Input: part model. Units: mm. Frame: model coordinates. Face numbers are marked on the shaded views. A direction names the side the tool comes from. Coordinates: 2 decimals unless noted, no trailing zeros. Write each loop counter-clockwise with the first axis right and the second up, starting at its lowest first coordinate (ties: lowest second). Pieces come first, ordered by that corner, then holes.
1) Set-up query: the marked faces 5, 6, 7, 8 and 9. Return all of +Z, -Z, +X, -X, +Y, -Y with unobstructed straight access to the full face (end or side cutting, diameter ignored); none if empty.
2) Section query A-A (z = 2). State how many separate pieces and enclosed holes the cut face has, then the cut area to 3 significant figures.
3) Section query C-C (y = 65.75). Output: boundary loops of the cut face in (x, z), then the cut area to 3 significant figures.
4) Draft query along Y for the marked faces 1, 2, 3 and 4. Return one class per face: pulls with the +Y half, pulls with the -Y half, needs draft (parallel to the pull), parting line crosses it, or undercut.
5) Line query: L1, parallel to Z at x = 19.25, y = 55.75; L2, parallel to Z at x = 23, y = 59.5; L3, parallel to Z at x = 30, y = 65. Output: solid intervals per line, ascending.
6) Section query D-D (x = 24). Output: boundary loops of the cut face in (y, z).
7) Pin query (flat end, axial travel): pin 1 Ø0.8 at (x, y) = (29.5, 54.5) entering from -Z; pin 2 Ø6 at (x, z) = (26.5, 2) entering from +Y; pin 3 Ø4 at (x, z) = (20.5, 2) entering from +Y. Return the tip coordinate at first contact, or that it passes through.
8) Section query B-B (z = -3). Output: boundary loops of the cut face in (x, y), then the cut area to 3 significant figures.
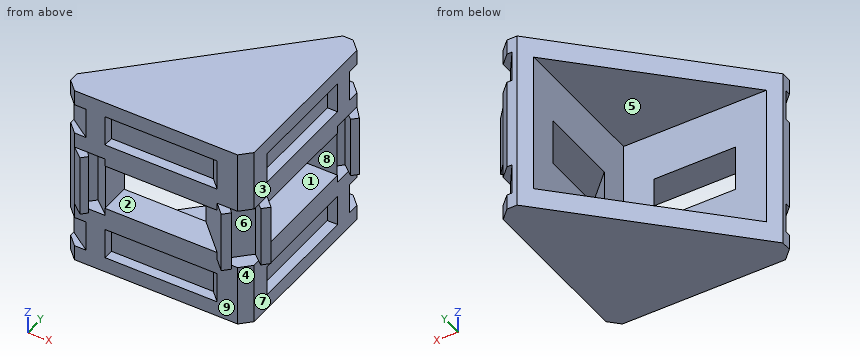
from build123d import *

# Parameters (mm, degrees)
EXTRUDE_1_DEPTH     = 6
EXTRUDE_1_2_DEPTH   = 6
EXTRUDE_1_3_DEPTH   = 6
EXTRUDE_2_DEPTH     = 4
EXTRUDE_3_DEPTH     = 2
EXTRUDE_4_DEPTH     = 0.75
EXTRUDE_5_DEPTH     = 0.75
CUT_EXTRUDE_2_DEPTH = 3
CUT_EXTRUDE_3_DEPTH = 3
CUT_EXTRUDE_4_DEPTH = 3
CUT_EXTRUDE_5_DEPTH = 3
CHAMFER_1_SIZE      = 1


with BuildPart() as part:
    # Sketch 1 → Extrude 1 (new body)
    with BuildSketch(Plane.XY):
        Polygon((32.591759834, 56.594303521), (33.206070874, 57.208614562), (29.145410702, 61.269274733), (29.145410702, 58.269274733), (26.145410702, 58.269274733), (30.206070874, 54.208614562), (30.820381914, 54.822925602), (29.852517484, 55.976381515), (31.438303921, 57.562167952), align=None)
    extrude(amount=EXTRUDE_1_DEPTH)



with BuildPart() as body_2:
    # Sketch 1 → Extrude 1 2 (new body)
    with BuildSketch(Plane.XY):
        Polygon((18.145410702, 55.352855481), (18.145410702, 58.269274733), (15.145410702, 58.269274733), (14.145410702, 57.269274733), (14.145410702, 56.269274733), (15.145410702, 55.269274733), (16.298866615, 54.301410302), (16.820381914, 54.822925602), (15.852517484, 55.976381515), (16.559624265, 56.683488296), align=None)
    extrude(amount=EXTRUDE_1_2_DEPTH)


with BuildPart() as body_3:
    # Sketch 1 → Extrude 1 3 (new body)
    with BuildSketch(Plane.XY):
        Polygon((31.438303921, 71.562167952), (32.591759834, 70.594303521), (33.113275133, 71.115818821), (32.145410702, 72.269274733), (31.145410702, 73.269274733), (30.145410702, 73.269274733), (29.145410702, 72.269274733), (29.145410702, 69.269274733), (32.061829955, 69.269274733), (30.73119714, 70.855061171), align=None)
    extrude(amount=EXTRUDE_1_3_DEPTH)


with BuildPart() as part_1:
    add(part.part)

    add(body_2.part)  # Extrude 2 merges body 2

    add(body_3.part)  # Extrude 2 merges body 3
    # Sketch 2 → Extrude 2 (add)
    with BuildSketch(Plane.XY.offset(6)):
        Polygon((30.145410702, 73.269274733), (31.145410702, 73.269274733), (32.145410702, 72.269274733), (32.145410702, 55.269274733), (15.145410702, 55.269274733), (14.145410702, 56.269274733), (14.145410702, 57.269274733), (15.145410702, 58.269274733), (29.145410702, 58.269274733), (29.145410702, 72.269274733), align=None)
    extrude_2 = extrude(amount=EXTRUDE_2_DEPTH)

    # Mirror 1: Extrude 2 across plane
    add(extrude_2.mirror(Plane(origin=(0, 0, 3), x_dir=(1, 0, 0), z_dir=(0, 0, -1))))

    # Sketch 3 → Extrude 3 (add)
    with BuildSketch(Plane.XY.offset(10)):
        Polygon((30.145410702, 73.269274733), (31.145410702, 73.269274733), (32.145410702, 72.269274733), (32.145410702, 55.269274733), (15.145410702, 55.269274733), (14.145410702, 56.269274733), (14.145410702, 57.269274733), align=None)
    extrude_3 = extrude(amount=EXTRUDE_3_DEPTH)

    # Mirror 2: Extrude 3 across plane
    add(extrude_3.mirror(Plane(origin=(0, 0, 3), x_dir=(1, 0, 0), z_dir=(0, 0, -1))))

    # Sketch 4 → Extrude 4 (add)
    with BuildSketch(Plane.XY):
        Polygon((29.145410702, 69.269274733), (32.145410702, 69.269274733), (32.145410702, 58.269274733), (29.145410702, 61.269274733), align=None)
    extrude_4 = extrude(amount=EXTRUDE_4_DEPTH)

    # Mirror 3: Extrude 4 across plane
    add(extrude_4.mirror(Plane(origin=(0, 0, 3), x_dir=(1, 0, 0), z_dir=(0, 0, -1))))

    # Sketch 5 → Extrude 5 (add)
    with BuildSketch(Plane.XY):
        Polygon((26.145410702, 58.269274733), (18.145410702, 58.269274733), (18.145410702, 55.269274733), (29.145410702, 55.269274733), align=None)
    extrude_5 = extrude(amount=EXTRUDE_5_DEPTH)

    # Mirror 4: Extrude 5 across plane
    add(extrude_5.mirror(Plane(origin=(0, 0, 3), x_dir=(1, 0, 0), z_dir=(0, 0, -1))))

    # Sketch 7 → Cut-Extrude 2 (cut)
    with BuildSketch(Plane(origin=(0, 0, -4.5), x_dir=(-1, 0, 0), z_dir=(0, 0, -1))):
        Polygon((-32.145410702, 69.269274733), (-31.145410702, 69.269274733), (-31.145410702, 59.269274733), (-32.145410702, 58.269274733), align=None)
    cut_extrude_2 = extrude(amount=-CUT_EXTRUDE_2_DEPTH, mode=Mode.SUBTRACT)

    # Sketch 8 → Cut-Extrude 3 (cut)
    with BuildSketch(Plane(origin=(0, 0, -4.5), x_dir=(-1, 0, 0), z_dir=(0, 0, -1))):
        Polygon((-18.145410702, 55.269274733), (-18.145410702, 56.269274733), (-28.145410702, 56.269274733), (-29.145410702, 55.269274733), align=None)
    cut_extrude_3 = extrude(amount=-CUT_EXTRUDE_3_DEPTH, mode=Mode.SUBTRACT)

    # Mirror 5: Cut-Extrude 2, Cut-Extrude 3 across plane
    add(cut_extrude_2.mirror(Plane(origin=(0, 0, 3), x_dir=(1, 0, 0), z_dir=(0, 0, -1))), mode=Mode.SUBTRACT)
    add(cut_extrude_3.mirror(Plane(origin=(0, 0, 3), x_dir=(1, 0, 0), z_dir=(0, 0, -1))), mode=Mode.SUBTRACT)

    # Sketch 9 → Cut-Extrude 4 (cut)
    with BuildSketch(Plane(origin=(0, 0, -4.5), x_dir=(-1, 0, 0), z_dir=(0, 0, -1))):
        Polygon((-30.645410702, 73.269274733), (-32.145410702, 71.127052723), (-32.145410702, 72.269274733), (-31.145410702, 73.269274733), align=None)
    cut_extrude_4 = extrude(amount=-CUT_EXTRUDE_4_DEPTH, mode=Mode.SUBTRACT)

    # Sketch 10 → Cut-Extrude 5 (cut)
    with BuildSketch(Plane(origin=(0, 0, -4.5), x_dir=(-1, 0, 0), z_dir=(0, 0, -1))):
        Polygon((-14.145410702, 56.769274733), (-16.287632713, 55.269274733), (-15.145410702, 55.269274733), (-14.145410702, 56.269274733), align=None)
    cut_extrude_5 = extrude(amount=-CUT_EXTRUDE_5_DEPTH, mode=Mode.SUBTRACT)

    # Mirror 6: Cut-Extrude 4, Cut-Extrude 5 across plane
    add(cut_extrude_4.mirror(Plane(origin=(0, 0, 3), x_dir=(1, 0, 0), z_dir=(0, 0, -1))), mode=Mode.SUBTRACT)
    add(cut_extrude_5.mirror(Plane(origin=(0, 0, 3), x_dir=(1, 0, 0), z_dir=(0, 0, -1))), mode=Mode.SUBTRACT)

    # Chamfer 1
    chamfer_1_edges = [part_1.edges().sort_by_distance(p)[0] for p in [
        (32.145410702, 55.269274733, -3),
        (32.145410702, 55.269274733, 9),
    ]]
    chamfer(chamfer_1_edges, length=CHAMFER_1_SIZE)


solid = part_1.part
Answer:
1. face 5: -X, +Y
1. face 6: none
1. face 7: -Z, +X
1. face 8: +X, -X
1. face 9: -Z, -Y
2. separate pieces: 3
2. enclosed holes: 0
2. area: 36.5 mm2
3. outline: (22.63, -6) - (32.15, -6) - (32.15, -4.5) - (31.15, -4.5) - (31.15, -1.5) - (32.15, -1.5) - (32.15, 0.75) - (29.15, 0.75) - (29.15, -4) - (22.63, -4) - close; (22.63, 10) - (29.15, 10) - (29.15, 5.25) - (32.15, 5.25) - (32.15, 7.5) - (31.15, 7.5) - (31.15, 10.5) - (32.15, 10.5) - (32.15, 12) - (22.63, 12) - close
3. area: 60.6 mm2
4. face 1: undercut
4. face 2: needs draft
4. face 3: undercut
4. face 4: pulls with the -Y half
5. L1: z = -6 to -4.5, -1.5 to 0.75, 5.25 to 7.5, 10.5 to 12
5. L2: z = -6 to -4, 10 to 12
5. L3: z = -6 to 0.75, 5.25 to 12
6. outline: (55.27, -6) - (67.12, -6) - (67.12, -4) - (58.27, -4) - (58.27, 0.75) - (55.27, 0.75) - (55.27, -1.5) - (56.27, -1.5) - (56.27, -4.5) - (55.27, -4.5) - close; (55.27, 5.25) - (58.27, 5.25) - (58.27, 10) - (67.12, 10) - (67.12, 12) - (55.27, 12) - (55.27, 10.5) - (56.27, 10.5) - (56.27, 7.5) - (55.27, 7.5) - close
7. pin 1: stops at z = 0
7. pin 2: stops at y = 72.62
7. pin 3: stops at y = 58.27
8. outline: (14.15, 56.77) - (16.29, 55.27) - (18.15, 55.27) - (18.15, 56.27) - (28.15, 56.27) - (29.15, 55.27) - (31.15, 55.27) - (32.15, 56.27) - (32.15, 58.27) - (31.15, 59.27) - (31.15, 69.27) - (32.15, 69.27) - (32.15, 71.13) - (30.65, 73.27) - (30.15, 73.27) - (29.15, 72.27) - (29.15, 58.27) - (15.15, 58.27) - (14.15, 57.27) - close
8. area: 73.3 mm2
